Part model, mm, in its own coordinate system. A direction names the side the tool comes from. Give positions to 0.01 mm unless a question says otherwise; leave off trailing zeros. Write each loop counter-clockwise with the first axis right and the second up, starting at its lowest first coordinate (ties: lowest second). Pieces come first, ordered by that corner, then holes. Notation, with made-up numbers: M 22.5,21 L 44.5,21 A14 cw 44.5,26 Z; hole C 45.25,87.25 d6. An arc over 180 degrees is marked long. Use a Markdown table: item, result.
Autodesk Inventor part; units mm, degrees
ref_plane "YZ Plane" through (0, 0, 0) normal (1, 0, 0) x (0, 1, 0)
ref_plane "XZ Plane" through (0, 0, 0) normal (0, 1, 0) x (-1, 0, 0)
ref_plane "XY Plane" through (0, 0, 0) normal (0, 0, 1) x (1, 0, 0)
sketch "Sketch1" plane through (0, 0, 0) normal (0, 0, 1) x (1, 0, 0)
  arc A0 (55, 0) -> (-55, 0) centre (0, 0) ccw
  line L0 (-55, 0) -> (55, 0)
  dimension "d0" = 55
  dimension "d1" = 110
revolve "Revolution1" add sketch "Sketch1" angle 180 about axis through (-55, 0, 0) along (-1, 0, 0)
sketch "Sketch2" plane through (0, 0, 0) normal (0, 0, 1) x (1, 0, 0)
  circle A0 centre (0, 0) radius 20
  dimension "d9" = 40
sketch "Sketch3" plane through (0, 0, 0) normal (0, 0, 1) x (1, 0, 0)
  line L0 (-34.2608, -17.3432) -> (-41.496, -17.3432)
  line L1 (-41.496, -17.3432) -> (-41.496, 17.3432)
  line L2 (-41.496, 17.3432) -> (-34.2608, 17.3432)
  line L3 (-34.2608, 17.3432) -> (-34.2608, -17.3432)
  line L4 (-34.2608, -17.3432) -> (-41.496, 17.3432) construction
  line L5 (-41.496, -17.3432) -> (-34.2608, 17.3432) construction
  line L6 (43.1984, -17.3432) -> (31.7072, -17.3432)
  line L7 (31.7072, -17.3432) -> (31.7072, 17.3432)
  line L8 (31.7072, 17.3432) -> (43.1984, 17.3432)
  line L9 (43.1984, 17.3432) -> (43.1984, -17.3432)
  line L10 (43.1984, -17.3432) -> (31.7072, 17.3432) construction
  line L11 (31.7072, -17.3432) -> (43.1984, 17.3432) construction
  point P0 (0, 0)
  point P1 (-37.8784, 0)
  point P2 (37.4528, 0)
extrude "Extrusion1" cut sketch "Sketch3" against normal blind 55
sketch "Sketch4" plane through (0, 0, 0) normal (0, 0, 1) x (1, 0, 0)
  line L0 (0, 35.7372) -> (-6.4528, 39.4627)
  line L1 (-6.4528, 39.4627) -> (-6.4528, 46.9137)
  line L2 (-6.4528, 46.9137) -> (0, 50.6392)
  line L3 (0, 50.6392) -> (6.4528, 46.9137)
  line L4 (6.4528, 46.9137) -> (6.4528, 39.4627)
  line L5 (6.4528, 39.4627) -> (0, 35.7372)
  line L6 (0, -31.5978) -> (7.6477, -36.0132)
  line L7 (7.6477, -36.0132) -> (7.6477, -44.844)
  line L8 (7.6477, -44.844) -> (0, -49.2594)
  line L9 (0, -49.2594) -> (-7.6477, -44.844)
  line L10 (-7.6477, -44.844) -> (-7.6477, -36.0132)
  line L11 (-7.6477, -36.0132) -> (0, -31.5978)
  point P0 (0, 0)
  point P1 (0, 43.1882)
  point P2 (0, -40.4286)
extrude "Extrusion2" cut sketch "Sketch4" against normal blind 55
extrude "Extrusion4" add sketch "Sketch2" along normal blind 30
properties material "Aluminum 6061"
1. Cut at B-B, the plane z = -13. Give the cut face in (x, y), then the cut area to 3 significant figures.
Findings below:
| item | result |
|---|---|
| outline | C 0,0 d106.88; hole M -41.5,-17.34 L -34.26,-17.34 L -34.26,17.34 L -41.5,17.34 Z; hole M -7.65,-44.84 L 0,-49.26 L 7.65,-44.84 L 7.65,-36.01 L 0,-31.6 L -7.65,-36.01 Z; hole M -6.45,39.46 L 0,35.74 L 6.45,39.46 L 6.45,46.91 L 0,50.64 L -6.45,46.91 Z; hole M 31.71,-17.34 L 43.2,-17.34 L 43.2,17.34 L 31.71,17.34 Z |
| area | 7,980 mm2 |
2. Two-plate mould, pull along Y, no slides. Class faces 3 (the flat face through (7.648, -40, -20)), 4 (the cylindrical face through (-4.336, 19.524, 14.79)), 5 (the flat face through (0, 0, 30)): released by +Y, released by -Y, zero draft, split by the parting line, or undercut.
Findings below:
| item | result |
|---|---|
| face 3 | undercut |
| face 4 | split by the parting line |
| face 5 | zero draft |
3. Tool access for faces 1 (the flat face through (-1, -24, 0)), 2 (the flat face through (-41.496, 0, -18)): list every direction of +Z, -Z, +X, -X, +Y, -Y with a clear straight run to the whole face (end or side of a thin tool).
Findings below:
| item | result |
|---|---|
| face 1 | +Z |
| face 2 | +Z, -Z |
4. Drill centre lines: L1, parallel to X at y = -7, z = -15.5; L2, parallel to X at y = -0.5, z = -27; L3, parallel to X at y = -20.5, z = -12.5. Where is each one in solid material? Low to high.
Findings below:
| item | result |
|---|---|
| L1 | -52.3 to -41.5, -34.26 to 31.71, 43.2 to 52.3 |
| L2 | -47.91 to -41.5, -34.26 to 31.71, 43.2 to 47.91 |
| L3 | -49.48 to 49.48 |
5. Cut at C-C, the plane y = 14.5. Give the cut face in (x, z), then the cut area to 3 significant figures.
Findings below:
| item | result |
|---|---|
| outline | M -53.05,0 A53.05 ccw -41.5,-33.06 L -41.5,0 Z; M -34.26,-40.51 A53.05 ccw 31.71,-42.54 L 31.71,0 L 13.77,0 L 13.77,30 L -13.77,30 L -13.77,0 L -34.26,0 Z; M 43.2,-30.8 A53.05 ccw 53.05,0 L 43.2,0 Z |
| area | 4,550 mm2 |
6. Drop flat-ended pins along their axis: P1, Ø8, axis at x = -38.5, z = -28, coming from the +Y side; P2, Ø2, axis at y = 42, z = -24, coming from the +X side; P3, Ø8, axis at y = 44.5, z = -22, coming from the -X side; P4, Ø4, axis at y = -41, z = 2.5, coming from the +X side. Give the stop position or say it passes through.
Findings below:
| item | result |
|---|---|
| P1 | y = 33.52 |
| P2 | x = 27.94 |
| P3 | x = -30.69 |
| P4 | through |
7. Cut at D-D, the plane x = 12. Give the cut face in (y, z), then the cut area to 3 significant figures.
Findings below:
| item | result |
|---|---|
| outline | M -53.67,0 A53.67 ccw 53.67,0 L 16,0 L 16,30 L -16,30 L -16,0 Z |
| area | 5,490 mm2 |
8. Cut at A-A, the plane y = 0. Give the cut face in (x, z), then the cut area to 3 significant figures.
Findings below:
| item | result |
|---|---|
| outline | M -55,0 A55 ccw -41.5,-36.1 L -41.5,0 Z; M -34.26,-43.03 A55 ccw 31.71,-44.94 L 31.71,0 L 20,0 L 20,30 L -20,30 L -20,0 L -34.26,0 Z; M 43.2,-34.04 A55 ccw 55,0 L 43.2,0 Z |
| area | 5,200 mm2 |
